Check sheet for the modelled part. Datum: model origin and axes. Units: mm. A direction names the side the tool comes from. Coordinates: 2 decimals unless noted, no trailing zeros. Write each loop counter-clockwise with the first axis right and the second up, starting at its lowest first coordinate (ties: lowest second). Pieces come first, ordered by that corner, then holes. Notation, with made-up numbers: M 59.5,15 L 108.5,15 A16 cw 108.5,28 Z; hole C 12.5,-32.5 d7. An arc over 180 degrees is marked long. Answer as CSV lines item,"result". Start each with the question number.
Q1. Depth check by flat-ended pin: pin 1 Ø5.5 at (x, z) = (-25, 115) entering from -Y; pin 2 Ø2.5 at (y, z) = (9, 240.5) entering from +X; pin 3 Ø3.5 at (y, z) = (9, 115.5) entering from -X; pin 4 Ø2 at (x, z) = (25, 115) entering from -Y. Enter the tip coordinate at first touch or a pass-through.
Q2. Sectioned sample at B-B, the plane y = 8.5. Record the cut outline in (x, z).
Q3. Thickness scan on line 1 along Z through (x, y) = (25, 5.75); line 2 along X through (y, z) = (6, 115); line 3 along X through (y, z) = (6.55, 240). Record the ranges inside material, lowest first. Write a range as from..to.
Q4. Sectioned sample at A-A, the plane z = 240. Record the cut outline in (x, y).
Q5. Sectioned sample at C-C, the plane x = -13. Record the cut outline in (y, z).
Q6. Access from +Z, -Z, +X, -X, +Y, -Y to the whole of each face (thin tool, end or side, straight path). Record for faces 1 (the cylindrical face through (19.779, 6.037, 241.686)), 2 (the flat face through (-26.47, 8.52, 117.5)), 3 (the flat face through (0, 5.1, 240)).
Q7. Mould release check, pull along Z, two halves, no side actions. Record for faces 4 (the flat face through (-1, 5.1, 115)), 5 (the cylindrical face through (-20.221, 6.037, 241.686)), 6 (the flat face through (0, 3, 230)): pulls with the +Z half, pulls with the -Z half, needs draft (parallel to the pull), parting line crosses it, or undercut.
Q8. Sectioned sample at D-D, the plane z = 115. Record the cut outline in (x, y), then the cut area to 3 significant figures.
from build123d import *

# Parameters (mm, degrees)
SKETCH1_R           = 50
BOSS_EXTRUDE1_DEPTH = 10
SKETCH2_R           = 20
CUT_EXTRUDE1_DEPTH  = 5
CUT_EXTRUDE6_DEPTH  = 3
SKETCH8_R           = 1.7
CUT_EXTRUDE7_DEPTH  = 10
BOSS_EXTRUDE3_DEPTH = 10
SKETCH10_W          = 21
SKETCH10_H          = 41
CUT_EXTRUDE8_DEPTH  = 10
SKETCH11_W          = 21
SKETCH11_H          = 6.5
CUT_EXTRUDE9_DEPTH  = 1.5
SKETCH12_R          = 1.7
CUT_EXTRUDE10_DEPTH = 9
CUT_EXTRUDE11_DEPTH = 10
SKETCH15_W          = 131.735170003
SKETCH15_H          = 179.266555965
CUT_EXTRUDE12_DEPTH = 79
BOSS_EXTRUDE4_DEPTH = 4.9
SKETCH17_R          = 1.7
CUT_EXTRUDE13_DEPTH = 10
CUT_EXTRUDE14_DEPTH = 3
SKETCH19_W          = 78.571428572
SKETCH19_H          = 5.1
CUT_EXTRUDE15_DEPTH = 0.5
SKETCH20_W          = 92.611657501
SKETCH20_H          = 114.528704683
CUT_EXTRUDE16_DEPTH = 10
CUT_EXTRUDE17_DEPTH = 5.1
SKETCH22_R          = 1.7
CUT_EXTRUDE18_DEPTH = 5.1
CUT_EXTRUDE19_DEPTH = 3


with BuildPart() as part:
    # Sketch1 → Boss-Extrude1 (new body)
    with BuildSketch(Plane(origin=(0, 0, 0), x_dir=(1, 0, 0), z_dir=(0, 1, 0))):
        Circle(SKETCH1_R)
    extrude(amount=BOSS_EXTRUDE1_DEPTH)

    # Sketch2 → Cut-Extrude1 (cut)
    with BuildSketch(Plane(origin=(0, 10, 0), x_dir=(1, 0, 0), z_dir=(0, 1, 0))):
        Circle(SKETCH2_R)
    extrude(amount=-CUT_EXTRUDE1_DEPTH, mode=Mode.SUBTRACT)

    # Sketch7 → Cut-Extrude6 (cut)
    with BuildSketch(Plane.XZ):
        with BuildLine():
            ThreePointArc((-2.85, 14.726761355), (0, 15), (2.85, 14.726761355))
            Line((2.85, 14.726761355), (2.85, 16.645448267))
            Line((2.85, 16.645448267), (0, 18.290896534))
            Line((0, 18.290896534), (-2.85, 16.645448267))
            Line((-2.85, 16.645448267), (-2.85, 14.726761355))
        make_face()
        with BuildLine():
            Line((2.85, 13.354551733), (2.85, 14.726761355))
            ThreePointArc((2.85, 14.726761355), (0, 15), (-2.85, 14.726761355))
            Line((-2.85, 14.726761355), (-2.85, 13.354551733))
            Line((-2.85, 13.354551733), (0, 11.709103466))
            Line((0, 11.709103466), (2.85, 13.354551733))
        make_face()
        Polygon((-12.990381057, -4.209103466), (-15.840381057, -5.854551733), (-15.840381057, -9.145448267), (-12.990381057, -10.790896534), (-10.140381057, -9.145448267), (-10.140381057, -5.854551733), align=None)
        Polygon((15.840381057, -5.854551733), (12.990381057, -4.209103466), (10.140381057, -5.854551733), (10.140381057, -9.145448267), (12.990381057, -10.790896534), (15.840381057, -9.145448267), align=None)
    extrude(amount=-CUT_EXTRUDE6_DEPTH, mode=Mode.SUBTRACT)

    # Sketch8 → Cut-Extrude7 (cut)
    with BuildSketch(Plane.XZ):
        with Locations((0, 15)):
            Circle(SKETCH8_R)
        with Locations((12.990381057, -7.5)):
            Circle(SKETCH8_R)
        with Locations((-12.990381057, -7.5)):
            Circle(SKETCH8_R)
    extrude(amount=-CUT_EXTRUDE7_DEPTH, mode=Mode.SUBTRACT)


with BuildPart() as body_2:
    # Sketch9 → Boss-Extrude3 (new body)
    with BuildSketch(Plane.XZ):
        with BuildLine():
            Line((-50, 350), (-50, 0))
            ThreePointArc((-50, 0), (0, 50), (50, 0))
            Line((50, 0), (50, 350))
            Line((50, 350), (-50, 350))
        make_face()
    extrude(amount=-BOSS_EXTRUDE3_DEPTH)

    # Sketch10 → Cut-Extrude8 (cut)
    with BuildSketch(Plane.XZ):
        with Locations((0, 319.5)):
            Rectangle(SKETCH10_W, SKETCH10_H)
    extrude(amount=-CUT_EXTRUDE8_DEPTH, mode=Mode.SUBTRACT)

    # Sketch11 → Cut-Extrude9 (cut)
    with BuildSketch(Plane.XZ):
        with Locations((0, 343.25)):
            Rectangle(SKETCH11_W, SKETCH11_H)
        with Locations((0, 295.75)):
            Rectangle(SKETCH11_W, SKETCH11_H)
    extrude(amount=-CUT_EXTRUDE9_DEPTH, mode=Mode.SUBTRACT)

    # Sketch12 → Cut-Extrude10 (cut)
    with BuildSketch(Plane.XZ.offset(-1.5)):
        with Locations((-5, 343.75)):
            Circle(SKETCH12_R)
        with Locations((5, 343.75)):
            Circle(SKETCH12_R)
        with Locations((-5, 295.25)):
            Circle(SKETCH12_R)
        with Locations((5, 295.25)):
            Circle(SKETCH12_R)
    extrude(amount=-CUT_EXTRUDE10_DEPTH, mode=Mode.SUBTRACT)

    # Sketch13 → Cut-Extrude11 (cut)
    with BuildSketch(Plane.XZ):
        with BuildLine():
            Line((-50, 350), (-50, 0))
            ThreePointArc((-50, 0), (-49.817332452, 4.270057067), (-49.270664506, 8.5089141))
            Line((-49.270664506, 8.5089141), (-20, 350))
            Line((-20, 350), (-50, 350))
        make_face()
        with BuildLine():
            Line((20, 350), (49.270664506, 8.5089141))
            ThreePointArc((49.270664506, 8.5089141), (49.817332452, 4.270057067), (50, 0))
            Line((50, 0), (50, 350))
            Line((50, 350), (20, 350))
        make_face()
    extrude(amount=-CUT_EXTRUDE11_DEPTH, mode=Mode.SUBTRACT)


with BuildPart() as cut_extrude12_tool:
    # Sketch15 → Cut-Extrude12 (new body)
    with BuildSketch(Plane(origin=(0, 10, 0), x_dir=(1, 0, 0), z_dir=(0, 1, 0))):
        with Locations((-8.166136658, -35.366722018)):
            Rectangle(SKETCH15_W, SKETCH15_H)
    extrude(amount=-CUT_EXTRUDE12_DEPTH)


with BuildPart() as part_1:
    add(part.part)

    # Cut-Extrude12: cut by cut_extrude12_tool
    add(cut_extrude12_tool.part, mode=Mode.SUBTRACT)


with BuildPart() as body_2_1:
    add(body_2.part)

    # Cut-Extrude12: cut by cut_extrude12_tool
    add(cut_extrude12_tool.part, mode=Mode.SUBTRACT)

    # Sketch16 → Boss-Extrude4 (add)
    with BuildSketch(Plane(origin=(0, 10, 0), x_dir=(1, 0, 0), z_dir=(0, 1, 0))):
        Polygon((40.972386827, -105.322153681), (-40.972386827, -105.322153681), (-39.285714286, -125), (39.285714286, -125), align=None)
    extrude(amount=-BOSS_EXTRUDE4_DEPTH)

    # Sketch17 → Cut-Extrude13 (cut)
    with BuildSketch(Plane.XZ.offset(-5.1)):
        with Locations((-25, 115)):
            Circle(SKETCH17_R)
        with Locations((25, 115)):
            Circle(SKETCH17_R)
    extrude(amount=-CUT_EXTRUDE13_DEPTH, mode=Mode.SUBTRACT)

    # Sketch18 → Cut-Extrude14 (cut)
    with BuildSketch(Plane(origin=(0, 10, 0), x_dir=(1, 0, 0), z_dir=(0, 1, 0))):
        Polygon((-25, -111.651368439), (-27.9, -113.325684219), (-27.9, -116.674315781), (-25, -118.348631561), (-22.1, -116.674315781), (-22.1, -113.325684219), align=None)
        Polygon((22.1, -113.325684219), (25, -111.651368439), (27.9, -113.325684219), (27.9, -116.674315781), (25, -118.348631561), (22.1, -116.674315781), align=None)
    extrude(amount=-CUT_EXTRUDE14_DEPTH, mode=Mode.SUBTRACT)

    # Sketch19 → Cut-Extrude15 (cut)
    with BuildSketch(Plane(origin=(0, 0, 125), x_dir=(-1, 0, 0), z_dir=(0, 0, -1))):
        with Locations((0, 2.55)):
            Rectangle(SKETCH19_W, SKETCH19_H)
    extrude(amount=-CUT_EXTRUDE15_DEPTH, mode=Mode.SUBTRACT)

    # Sketch20 → Cut-Extrude16 (cut)
    with BuildSketch(Plane.XZ):
        with Locations((0.685731612, 307.264352342)):
            Rectangle(SKETCH20_W, SKETCH20_H)
    extrude(amount=-CUT_EXTRUDE16_DEPTH, mode=Mode.SUBTRACT)

    # Sketch21 → Cut-Extrude17 (cut)
    with BuildSketch(Plane.XZ):
        Polygon((-28.571428571, 250), (-30.285714286, 230), (30.285714286, 230), (28.571428571, 250), align=None)
    extrude(amount=-CUT_EXTRUDE17_DEPTH, mode=Mode.SUBTRACT)

    # Sketch22 → Cut-Extrude18 (cut)
    with BuildSketch(Plane.XZ.offset(-5.1)):
        with Locations((-20, 240)):
            Circle(SKETCH22_R)
        with Locations((20, 240)):
            Circle(SKETCH22_R)
    extrude(amount=-CUT_EXTRUDE18_DEPTH, mode=Mode.SUBTRACT)

    # Sketch23 → Cut-Extrude19 (cut)
    with BuildSketch(Plane(origin=(0, 10, 0), x_dir=(1, 0, 0), z_dir=(0, 1, 0))):
        Polygon((-20, -236.651368439), (-22.9, -238.325684219), (-22.9, -241.674315781), (-20, -243.348631561), (-17.1, -241.674315781), (-17.1, -238.325684219), align=None)
        Polygon((17.1, -238.325684219), (20, -236.651368439), (22.9, -238.325684219), (22.9, -241.674315781), (20, -243.348631561), (17.1, -241.674315781), align=None)
    extrude(amount=-CUT_EXTRUDE19_DEPTH, mode=Mode.SUBTRACT)


solid = body_2_1.part
Output:
1,pin 1,"stops at y = 5.1"
1,pin 2,"stops at x = 29.49"
1,pin 3,"stops at x = -40.25"
1,pin 4,"passes through"
2,outline,"M -40.97,105.32 L 40.97,105.32 L 28.57,250 L -28.57,250 Z; hole M -27.9,113.33 L -25,111.65 L -22.1,113.33 L -22.1,116.67 L -25,118.35 L -27.9,116.67 Z; hole M -22.9,238.33 L -20,236.65 L -17.1,238.33 L -17.1,241.67 L -20,243.35 L -22.9,241.67 Z; hole M 17.1,238.33 L 20,236.65 L 22.9,238.33 L 22.9,241.67 L 20,243.35 L 17.1,241.67 Z; hole M 22.1,113.33 L 25,111.65 L 27.9,113.33 L 27.9,116.67 L 25,118.35 L 22.1,116.67 Z"
3,line 1,"z = 105.32..113.3, 116.7..250"
3,line 2,"x = -40.14..-26.7, -23.3..23.3, 26.7..40.14"
3,line 3,"x = -29.43..-21.7, -18.3..18.3, 21.7..29.43"
4,outline,"M -29.43,5.1 L -21.7,5.1 L -21.7,7 L -22.9,7 L -22.9,10 L -29.43,10 Z; M -18.3,5.1 L 18.3,5.1 L 18.3,7 L 17.1,7 L 17.1,10 L -17.1,10 L -17.1,7 L -18.3,7 Z; M 21.7,5.1 L 29.43,5.1 L 29.43,10 L 22.9,10 L 22.9,7 L 21.7,7 Z"
5,outline,"M 0,125.5 L 5.1,125.5 L 5.1,105.32 L 10,105.32 L 10,250 L 5.1,250 L 5.1,230 L 0,230 Z"
6,face 1,"+Y, -Y"
6,face 2,"+Y"
6,face 3,"+Z, +X, -X, -Y"
7,face 4,"needs draft"
7,face 5,"undercut"
7,face 6,"pulls with the +Z half"
8,outline,"M -40.14,5.1 L -26.7,5.1 L -26.7,7 L -27.9,7 L -27.9,10 L -40.14,10 Z; M -23.3,5.1 L 23.3,5.1 L 23.3,7 L 22.1,7 L 22.1,10 L -22.1,10 L -22.1,7 L -23.3,7 Z; M 26.7,5.1 L 40.14,5.1 L 40.14,10 L 27.9,10 L 27.9,7 L 26.7,7 Z"
8,area,"346 mm^2"
